Autodesk Inventor part; units mm, degrees
ref_plane "YZ Plane" through (0, 0, 0) normal (1, 0, 0) x (0, 1, 0)
ref_plane "XZ Plane" through (0, 0, 0) normal (0, 1, 0) x (-1, 0, 0)
ref_plane "XY Plane" through (0, 0, 0) normal (0, 0, 1) x (1, 0, 0)
sketch "Sketch1" plane through (0, 0, 0) normal (0, 1, 0) x (-1, 0, 0)
  line L0 (170, 50) -> (-170, 50)
  line L1 (-170, 50) -> (-170, -50)
  line L2 (-170, -50) -> (170, -50)
  line L3 (170, -50) -> (170, 50)
  line L4 (170, 50) -> (-170, -50) construction
  line L5 (-170, 50) -> (170, -50) construction
  point P0 (0, 0)
  dimension "d0" = 340
  dimension "d1" = 100
extrude "Extrusion1" add sketch "Sketch1" along normal mid plane 3.125
fillet "Fillet1" radius 10 4 edges at (-170, 0, 50) (-170, 0, -50) (170, 0, -50) (170, 0, 50)
sketch "Sketch2" plane through (0, 1.5625, 0) normal (0, 1, 0) x (1, 0, 0)
  arc A0 (160, -50) -> (170, -40) centre (160, -40) ccw
  line L0 (160, 50) -> (-160, 50)
  arc A1 (-160, 50) -> (-170, 40) centre (-160, 40) ccw
  line L1 (-160, -50) -> (160, -50)
  line L2 (170, -40) -> (170, 40)
  arc A2 (170, 40) -> (160, 50) centre (160, 40) ccw
  line L3 (-170, 40) -> (-170, -40)
  arc A3 (-170, -40) -> (-160, -50) centre (-160, -40) ccw
  point P0 (0, 0)
  dimension "d0" = 340
  dimension "d6" = 10
  dimension "d14" = 10
hole "Hole1" at (-160, 1.5625, 40) direction (0, -1, 0) diameter 5.5118 end through all
mirror "Mirror1" about plane through (0, 0, 0) normal (0, 0, 1) of "Hole1"
mirror "Mirror2" about plane through (0, 0, 0) normal (1, 0, 0) of "Hole1", "Mirror1"
equation "\"d1\" = suppourtPlateLength"
equation "\"d2\" = acrylicThickness"
equation "\"suppourtPlateLength\" = 100"
equation "\"acrylicThickness\" = 3.125"
properties part number "supportPlate" material "ABS Plastic"
Geometry check sheet. Reference: the model listing, model coordinates, mm. Give positions to 0.01 mm unless a question says otherwise; leave off trailing zeros.
(1) Release check for a two-part mould opening along X. For faces 1 (the cylindrical face through (-167.15, 0.02, 46.99)), 2 (the cylindrical face through (-162.732, -0.022, 39.641)), 3 (the flat face through (2, -1.562, 1)) record: released by +X, released by -X, zero draft, split by the parting line, or undercut.
From the geometry:
face 1: released by -X
face 2: undercut
face 3: zero draft
(2) Thickness scan on L1, parallel to X at y = -0.35, z = 40; L2, parallel to Z at x = 160, y = -0.55; L3, parallel to X at y = -0.5, z = 41.5. Record the ranges inside material, lowest first.
From the geometry:
L1: x = -170 to -162.76, -157.24 to 157.24, 162.76 to 170
L2: z = -50 to -42.76, -37.24 to 37.24, 42.76 to 50
L3: x = -169.89 to -162.31, -157.69 to 157.69, 162.31 to 169.89
(3) Depth check by flat-ended pin: pin 1 Ø4.5 at (x, z) = (-160, 40) entering from +Y. Enter the tip coordinate at first touch or a pass-through.
From the geometry:
pin 1: passes through
